The listing builds one solid part. Answer for the finished solid, in the listing's coordinates (mm). A direction names the side the tool comes from. Give positions to 0.01 mm unless a question says otherwise; leave off trailing zeros. Write each loop counter-clockwise with the first axis right and the second up, starting at its lowest first coordinate (ties: lowest second). Pieces come first, ordered by that corner, then holes. Notation, with made-up numbers: (74, 8) -> (117, 8) arc R17 cw to (117, 22) -> close; hole circle Ø11 at (-11, 9.25). An arc over 180 degrees is marked (long way). One line per question, with ' | ' between items.
from build123d import *

# Parameters (mm, degrees)
SKETCH_1_W      = 26.3
SKETCH_1_H      = 22
SKETCH_1_R      = 3
SKETCH_1_R_2    = 1.25
EXTRUDE_1_DEPTH = 2.1
FILLET_1_R      = 1


with BuildPart() as part:
    # 草图1 → 凸台-拉伸1 (new body)
    with BuildSketch(Plane(origin=(0, 0, 0), x_dir=(0, 0, -1), z_dir=(1, 0, 0))):
        Rectangle(SKETCH_1_W, SKETCH_1_H)
        with BuildLine():
            ThreePointArc((-6.8, -5.55), (-7.10753788, -6.29246212), (-7.85, -6.6))
            Line((-7.85, -6.6), (-10.15, -6.6))
            ThreePointArc((-10.15, -6.6), (-11.2, -5.55), (-10.15, -4.5))
            Line((-10.15, -4.5), (-10.15, -0.5))
            ThreePointArc((-10.15, -0.5), (-11.2, 0.55), (-10.15, 1.6))
            Line((-10.15, 1.6), (-7.85, 1.6))
            ThreePointArc((-7.85, 1.6), (-7.10753788, 1.29246212), (-6.8, 0.55))
            ThreePointArc((-6.8, 0.55), (-7.10753788, -0.19246212), (-7.85, -0.5))
            Line((-7.85, -0.5), (-7.85, -4.5))
            ThreePointArc((-7.85, -4.5), (-7.10753788, -4.80753788), (-6.8, -5.55))
        make_face(mode=Mode.SUBTRACT)
        with Locations((0, -4)):
            Circle(SKETCH_1_R, mode=Mode.SUBTRACT)
        with BuildLine():
            ThreePointArc((11.2, -5.55), (10.89246212, -6.29246212), (10.15, -6.6))
            Line((10.15, -6.6), (7.85, -6.6))
            ThreePointArc((7.85, -6.6), (6.8, -5.55), (7.85, -4.5))
            Line((7.85, -4.5), (7.85, -0.5))
            ThreePointArc((7.85, -0.5), (6.8, 0.55), (7.85, 1.6))
            Line((7.85, 1.6), (10.15, 1.6))
            ThreePointArc((10.15, 1.6), (10.89246212, 1.29246212), (11.2, 0.55))
            ThreePointArc((11.2, 0.55), (10.89246212, -0.19246212), (10.15, -0.5))
            Line((10.15, -0.5), (10.15, -4.5))
            ThreePointArc((10.15, -4.5), (10.89246212, -4.80753788), (11.2, -5.55))
        make_face(mode=Mode.SUBTRACT)
        with Locations((-11, 5.5)):
            Circle(SKETCH_1_R_2, mode=Mode.SUBTRACT)
        with BuildLine():
            Line((3, 5.9), (-3, 5.9))
            ThreePointArc((-3, 5.9), (-4.05, 4.85), (-5.1, 5.9))
            Line((-5.1, 5.9), (-5.1, 8.2))
            ThreePointArc((-5.1, 8.2), (-4.05, 9.25), (-3, 8.2))
            Line((-3, 8.2), (3, 8.2))
            ThreePointArc((3, 8.2), (4.05, 9.25), (5.1, 8.2))
            Line((5.1, 8.2), (5.1, 5.9))
            ThreePointArc((5.1, 5.9), (4.05, 4.85), (3, 5.9))
        make_face(mode=Mode.SUBTRACT)
        with Locations((11, 5.5)):
            Circle(SKETCH_1_R_2, mode=Mode.SUBTRACT)
    extrude(amount=EXTRUDE_1_DEPTH)

    # 圆角1
    fillet_1_edges = [part.edges().sort_by_distance(p)[0] for p in [
        (1.05, 11, 13.15),
        (1.05, 11, -13.15),
        (1.05, -11, -13.15),
        (1.05, -11, 13.15),
    ]]
    fillet(fillet_1_edges, radius=FILLET_1_R)


solid = part.part
Item 1: A tool of negligible diameter and unlimited length cuts with its end or side. For faces 1 (the face through (1, -5.6, 11.2)), 2 (the face through (1, 0, -13.15)), from which of +Z, -Z, +X, -X, +Y, -Y can it reach the whole face along a straight path? Write none if from no direction.
Answers below:
face 1: +X, -X | face 2: -Z, +X, -X, +Y, -Y
Item 2: Consider line 1 (Y direction, x = 0.85, z = 0); line 2 (Z direction, x = 1.8, y = -1.75); line 3 (Z direction, x = 1.8, y = 7.5). Determine where each line is inside the solid, lowest interval first. Write a range as [from, to].
Answers below:
line 1: [-11, -7], [-1, 5.9], [8.2, 11] | line 2: [-13.15, -10.15], [-7.85, -1.98], [1.98, 7.85], [10.15, 13.15] | line 3: [-13.15, -5.1], [5.1, 13.15]
Item 3: Find section D-D (z = -3.75). Write down the section's boundary in (x, y), then the cut area to 3 significant figures.
Answers below:
outline: (0, -11) -> (2.1, -11) -> (2.1, 4.89) -> (0, 4.89) -> close; (0, 9.21) -> (2.1, 9.21) -> (2.1, 11) -> (0, 11) -> close | area: 37.1 mm²
Item 4: Find section B-B (y = 5.5). Write down the section's boundary in (x, z), then the cut area to 3 significant figures.
Answers below:
outline: (0, -13.15) -> (2.1, -13.15) -> (2.1, -12.25) -> (0, -12.25) -> close; (0, -9.75) -> (2.1, -9.75) -> (2.1, -5.02) -> (0, -5.02) -> close; (0, -3.08) -> (2.1, -3.08) -> (2.1, 3.08) -> (0, 3.08) -> close; (0, 5.02) -> (2.1, 5.02) -> (2.1, 9.75) -> (0, 9.75) -> close; (0, 12.25) -> (2.1, 12.25) -> (2.1, 13.15) -> (0, 13.15) -> close | area: 36.6 mm²
Item 5: Find section A-A (z = 9.25). Write down the section's boundary in (x, y).
Answers below:
outline: (0, -11) -> (2.1, -11) -> (2.1, -6.6) -> (0, -6.6) -> close; (0, 1.6) -> (2.1, 1.6) -> (2.1, 11) -> (0, 11) -> close
Item 6: Find section C-C (x = 1.55). Count the separate pieces of the cut face and the enclosed holes in it, then the cut area to 3 significant figures.
Answers below:
separate pieces: 1 | enclosed holes: 6 | area: 458 mm²
Item 7: A flat-ended cylindrical pin translates along its axis: pin 1 (4 mm diameter, centred on y = -5.5, z = 4.5, fed in from -X). Find the tip coordinate at first contact, or state that the pin passes through.
Answers below:
pin 1: x = 0
Item 8: Determine the mould class of faces 3 (the face through (1, -1, 0)), 4 (the face through (1.065, 10.699, 12.865)), 5 (the face through (2.1, 0, 0)) for opening direction Y: pulls with the +Y half, pulls with the -Y half, needs draft (parallel to the pull), parting line crosses it, or undercut.
Answers below:
face 3: undercut | face 4: pulls with the +Y half | face 5: needs draft
